Design review of the part built by this model. Coordinates are the model's own, in mm. A direction names the side the tool comes from. Coordinates: 2 decimals unless noted, no trailing zeros. Loops run counter-clockwise (first coordinate to the right, second up) from the corner with the lowest first, then second, coordinate; pieces in that order, holes last. Notation, with made-up numbers: M 26.25,15 L 42.25,15 A5 ccw 42.25,21 Z; hole C 75,26.5 d4. An arc over 180 degrees is marked long. Put each result on its own line as item: value. Start each with the question number.
(1) For faces 1 (the cylindrical face through (-4.1, 0.7, 12.8)), 2 (the flat face through (11.3, 1, 2)), 3 (the flat face through (0, 0.5, 7)), list the 3-axis set-ups (+Z, -Z, +X, -X, +Y, -Y) from which the entire face can be reached by the end or side of a thin tool; tool diameter is ignored.
(2) Take a section at A-A, the plane x = -3.5. Give the boundary of the cut face in (y, z), then the cut area to 3 significant figures.
(3) Take a section at D-D, the plane z = 0. Give the boundary of the cut face in (x, y), then the cut area to 4 significant figures.
(4) Take a section at B-B, the plane z = 4. Give the boundary of the cut face in (x, y), then the cut area to 3 significant figures.
(5) For probe 1 along X at (y, z) = (2.4, 11); probe 2 along X at (y, z) = (0.6, 4); probe 3 along Z at (x, y) = (5.75, 1.15), list the stretches that pass through material, from the lowest coordinate up. Write a range as [from, to].
(6) Take a section at C-C, the plane x = 9.8. Give the boundary of the cut face in (y, z).
(7) Clearance check with flat-ended pins moving along their axes: pin 1 (1.3 mm diameter, centred on x = -3.5, z = 12, fed in from -Y); pin 2 (1.6 mm diameter, centred on x = -3.5, z = -9.6, fed in from -Y); pin 3 (1 mm diameter, centred on x = 5.5, z = -8, fed in from +Y). State where each tip first meets the part, or that it passes through.
(8) The part is to be moulded in two halves that separate along X. For faces 4 (the cylindrical face through (9.532, 2.24, 10.353)), 5 (the flat face through (3, 3, 1.2)), 6 (the flat face through (-5, 1, 2)), say which applies: +X half, -X half, draft (parallel to the pull), parting line (faces both ways), or undercut.
```python
from build123d import *

# Parameters (mm, degrees)
SKETCH_1_W          = 16.3
SKETCH_1_H          = 31.2
EXTRUDE_1_DEPTH     = 3
CUT_EXTRUDE_START   = 3
SKETCH_1_3_R        = 3.05
SKETCH_1_3_R_2      = 2.55
SKETCH_1_3_R_3      = 1.05
CUT_EXTRUDE_1_DEPTH = 2.5
SKETCH_2_R          = 1
CUT_EXTRUDE_2_DEPTH = 1.5
SKETCH_2_3_R        = 0.7
CUT_EXTRUDE_3_DEPTH = 21.632256299


with BuildPart() as part:
    # 草图1 → 凸台-拉伸1 (new body)
    with BuildSketch(Plane(origin=(0, 0, 0), x_dir=(1, 0, 0), z_dir=(0, 1, 0))):
        with Locations((3.15, -1.4)):
            Rectangle(SKETCH_1_W, SKETCH_1_H)
    extrude(amount=EXTRUDE_1_DEPTH)

    # 草图1<3> → 切除-拉伸1 (cut)
    with BuildSketch(Plane(origin=(0, 0, 0), x_dir=(1, 0, 0), z_dir=(0, 1, 0)).offset(CUT_EXTRUDE_START)):
        with Locations(Location((0, 0, 0), (0, 0, 90))):
            Circle(SKETCH_1_3_R)
        with Locations(Location((4.7, -11, 0), (0, 0, 90))):
            Circle(SKETCH_1_3_R_2)
        with Locations(Location((-0.337099263, -6.891760594, 0), (0, 0, 90))):
            Circle(SKETCH_1_3_R_2)
        with Locations(Location((5.25646039, 8.152277238, 0), (0, 0, 90))):
            Circle(SKETCH_1_3_R_3)
    extrude(amount=-CUT_EXTRUDE_1_DEPTH, mode=Mode.SUBTRACT)

    # 草图2 → 切除-拉伸2 (cut)
    with BuildSketch(Plane.XZ):
        with Locations(Location((9.8, 11, 0), (0, 0, 270))):
            Circle(SKETCH_2_R)
        with Locations(Location((-3.5, 12, 0), (0, 0, 270))):
            Circle(SKETCH_2_R)
        with Locations(Location((6.3, 4, 0), (0, 0, 270))):
            Circle(SKETCH_2_R)
        with Locations(Location((-3.5, -9.6, 0), (0, 0, 270))):
            Circle(SKETCH_2_R)
    extrude(amount=-CUT_EXTRUDE_2_DEPTH, mode=Mode.SUBTRACT)

    # 草图2<3> → 切除-拉伸3 (cut, through all)
    with BuildSketch(Plane.XZ):
        with Locations(Location((9.8, 11, 0), (0, 0, 270))):
            Circle(SKETCH_2_3_R)
        with Locations(Location((-3.5, 12, 0), (0, 0, 270))):
            Circle(SKETCH_2_3_R)
        with Locations(Location((6.3, 4, 0), (0, 0, 270))):
            Circle(SKETCH_2_3_R)
        with Locations(Location((-3.5, -9.6, 0), (0, 0, 270))):
            Circle(SKETCH_2_3_R)
    extrude(amount=-CUT_EXTRUDE_3_DEPTH, mode=Mode.SUBTRACT)


solid = part.part
```
Computed values:
1. face 1: -Y
1. face 2: +Z, -Z, +X, +Y, -Y
1. face 3: +Y
2. outline: M 0,-14.2 L 3,-14.2 L 3,-10.3 L 1.5,-10.3 L 1.5,-10.6 L 0,-10.6 Z; M 0,-8.6 L 1.5,-8.6 L 1.5,-8.9 L 3,-8.9 L 3,11.3 L 1.5,11.3 L 1.5,11 L 0,11 Z; M 0,13 L 1.5,13 L 1.5,12.7 L 3,12.7 L 3,17 L 0,17 Z
2. area: 83.4 mm^2
3. outline: M -5,0 L 11.3,0 L 11.3,3 L 3.05,3 L 3.05,0.5 L -3.05,0.5 L -3.05,3 L -5,3 Z
3. area: 33.65 mm^2
4. outline: M -5,0 L 5.3,0 L 5.3,1.5 L 5.6,1.5 L 5.6,3 L -5,3 Z; M 7,1.5 L 7.3,1.5 L 7.3,0 L 11.3,0 L 11.3,3 L 7,3 Z
4. area: 43.8 mm^2
5. probe 1: x = [-5, 2.15], [7.25, 9.1], [10.5, 11.3]
5. probe 2: x = [-5, 5.3], [7.3, 11.3]
5. probe 3: z = [-14.2, -9.08], [-7.23, 3.16], [4.84, 8.68], [13.32, 17]
6. outline: M 0,-14.2 L 3,-14.2 L 3,10.3 L 1.5,10.3 L 1.5,10 L 0,10 Z; M 0,12 L 1.5,12 L 1.5,11.7 L 3,11.7 L 3,17 L 0,17 Z
7. pin 1: passes through
7. pin 2: stops at y = 1.5
7. pin 3: stops at y = 0.5
8. face 4: undercut
8. face 5: draft
8. face 6: -X half
